CAD build for the part. Positions are in the model's coordinates, mm. Face numbers are marked on the shaded views. A direction names the side the tool comes from. Coordinates: 2 decimals unless noted, no trailing zeros. Order: outer loops, then holes, each group sorted by start corner. A loop starts at its lowest first (then second) coordinate and runs counter-clockwise, first axis right, second up.
from build123d import *

# Parameters (mm, degrees)
F1_DEPTH       = 35
F3_DEPTH       = 1
F4_W           = 3
F4_H           = 2
F5_DEPTH       = 25
F7_D           = 2.5
F7_CBORE_D     = 6
F7_CBORE_DEPTH = 2


with BuildPart() as f1:
    # F0 (on Front) → F1 (new body)
    with BuildSketch(Plane.XZ):
        with BuildLine():
            Line((0, 0.75), (0, 0))
            Line((0, 0), (6, 0))
            Line((6, 0), (6, 1.5))
            Line((6, 1.5), (4.5, 1.5))
            Line((4.5, 1.5), (4.5, 3))
            Line((4.5, 3), (6, 3))
            Line((6, 3), (6, 4.5))
            Line((6, 4.5), (1.25, 4.5))
            Line((1.25, 4.5), (1.25, 2))
            ThreePointArc((1.25, 2), (0.8838834765, 1.1161165235), (0, 0.75))
        make_face()
    extrude(amount=F1_DEPTH)

    # F2: F1 across plane


with BuildPart() as f1_1:
    add(f1.part)
    add(f1.part.mirror(Plane.YZ))

    # F0 (on Front) → F3 (join)
    with BuildSketch(Plane.XZ):
        Polygon((6, 0), (0, 0), (-6, 0), (-6, -1), (6, -1), align=None)
    extrude(amount=F3_DEPTH)

    # F4 (on Right) → F5 (cut, symmetric)
    with BuildSketch(Plane.YZ):
        with Locations((-31.5, 1)):
            Rectangle(F4_W, F4_H)
    extrude(amount=F5_DEPTH, both=True, mode=Mode.SUBTRACT)

    # F7 (through all)
    with Locations(Plane(origin=(0, 0, 0), x_dir=(1, 0, 0), z_dir=(0, 0, -1))):
        with Locations((0, 10)):
            CounterBoreHole(F7_D / 2, F7_CBORE_D / 2, F7_CBORE_DEPTH)


solid = f1_1.part
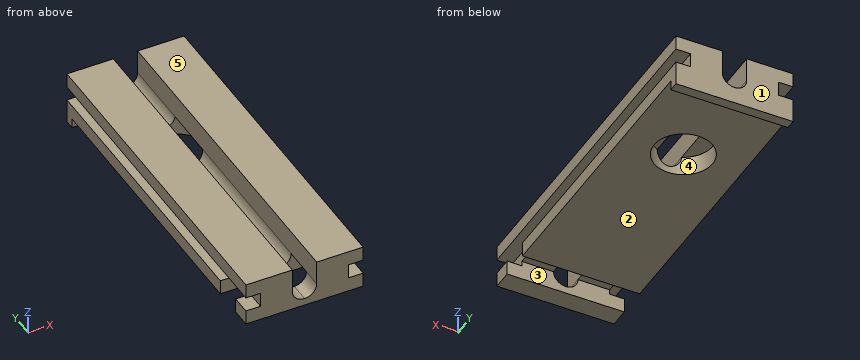
1) Drill centre lines: probe 1 along Y at (x, z) = (0, 0.6); probe 2 along X at (y, z) = (-9, 4.1); probe 3 along Y at (x, z) = (5.25, 0.3). Where is each one in solid material? Low to high.
2) Two-plate mould, pull along Y, no slides. Class the marked faces 1, 2 and 3: released by +Y, released by -Y, zero draft, split by the parting line, or undercut.
3) Slice it at B-B (z = 3.8). List the corners of the cut face in (x, y).
4) Pin check, flat tips, straight feed: P1, Ø1, axis at x = -3, y = -33.5, coming from the -Z side; P2, Ø1.5, axis at x = 3.5, y = -31, coming from the -Z side; P3, Ø0.5, axis at x = 1, z = -0.5, coming from the -Y side; P4, Ø1, axis at x = 0.5, z = 1.5, coming from the -Y side. Stop position of each tip, or through.
5) Which spindle directions (+Z, -Z, +X, -X, +Y, -Y) get a long thin tool onto all of the face, cutting with end or side? Do the marked faces 4 and 5. Say none if no direction does.
6) Slice it at C-C (z = 1.05). List the corners of the cut face in (x, y), plus the area to 3 significant figures.
7) Slice it at D-D (x = -0.75). List the corners of the cut face in (y, z).
8) Slice it at A-A (y = -32). List the corners of the cut face in (x, z), plus the area to 4 significant figures.
Worked out:
1. probe 1: y = -35 to -33, -30 to -13, -7 to 0
1. probe 2: x = -6 to -1.25, 1.25 to 6
1. probe 3: y = -35 to -33, -30 to 0
2. face 1: released by +Y
2. face 2: zero draft
2. face 3: undercut
3. outline: (-6, -35) - (-1.25, -35) - (-1.25, 0) - (-6, 0) - close; (1.25, -35) - (6, -35) - (6, 0) - (1.25, 0) - close
4. P1: stops at z = 0
4. P2: stops at z = 2
4. P3: stops at y = -1
4. P4: passes through
5. face 4: -Z
5. face 5: +Z, +X, -X, +Y, -Y
6. outline: (-6, -35) - (-0.81, -35) - (-0.81, -33) - (-6, -33) - close; (-6, -30) - (-0.81, -30) - (-0.81, -12.89) arc R3 cw to (-0.81, -7.11) - (-0.81, 0) - (-6, 0) - close; (0.81, -35) - (6, -35) - (6, -33) - (0.81, -33) - close; (0.81, -30) - (6, -30) - (6, 0) - (0.81, 0) - (0.81, -7.11) arc R3 cw to (0.81, -12.89) - close
6. area: 313 mm2
7. outline: (-35, 0) - (-33, 0) - (-33, 1) - (-35, 1) - close; (-30, 0) - (-12.9, 0) - (-12.9, 1) - (-30, 1) - close; (-7.1, 0) - (-1, 0) - (-1, -1) - (0, -1) - (0, 1) - (-7.1, 1) - close
8. outline: (-6, 3) - (-4.5, 3) - (-4.5, 2) - (-1.25, 2) - (-1.25, 4.5) - (-6, 4.5) - close; (1.25, 2) - (4.5, 2) - (4.5, 3) - (6, 3) - (6, 4.5) - (1.25, 4.5) - close
8. area: 20.75 mm2
